Build history of the part. All positions in model axes, mm. Face numbers are marked on the shaded views. A direction names the side the tool comes from. Give positions to 0.01 mm unless a question says otherwise; leave off trailing zeros. Order: outer loops, then holes, each group sorted by start corner. A loop starts at its lowest first (then second) coordinate and runs counter-clockwise, first axis right, second up. Notation, with made-up numbers: (81, 23) - (97, 23) arc R33 ccw to (97, 56) - close; hole circle Ø8 at (33, 7). An arc over 180 degrees is marked (long way). Use a Markdown table: item, result. Add a question column.
(1) Flat gauge pins, fed straight in: pin 1 (6 mm diameter, centred on x = -6.5, z = 0, fed in from +Y); pin 2 (0.6 mm diameter, centred on x = 17.5, y = 2.5, fed in from +Z); pin 3 (1.2 mm diameter, centred on x = -20.75, z = -7.75, fed in from -Y); pin 4 (1.6 mm diameter, centred on x = 20.5, y = 4.5, fed in from -Z). Where does each tip first touch, or does it go through?
(2) Slice it at A-A (z = 7.75). Write the cut outline in (x, y).
(3) Wall check: line 1 (Z direction, x = 20.75, y = 1.25); line 2 (X direction, y = 0.35, z = 7.75); line 3 (Y direction, x = -18.5, z = 3.5). Give the ranges that are in metal, low to high.
(4) Slice it at B-B (x = -20.75). Write the cut outline in (y, z), then the cut area to 3 significant figures.
(5) Slice it at D-D (z = 1.5). Write the cut outline in (x, y), then the cut area to 3 significant figures.
(6) Which spindle directions (+Z, -Z, +X, -X, +Y, -Y) get a long thin tool onto all of the face, cutting with end or side? Do the marked faces 1 and 2. Say none if no direction does.
(7) Slice it at C-C (x = 16). Write the cut outline in (y, z), then the cut area to 3 significant figures.
from build123d import *

# Parameters (mm, degrees)
SCHIZZO1_W                   = 44
SCHIZZO1_H                   = 18
ESTRUSIONE_ESTRUSIONE1_DEPTH = 1.5
SCHIZZO2_R                   = 0.75
TAGLIO_ESTRUSIONE1_DEPTH     = 1.5
SCHIZZO4_W                   = 10
SCHIZZO4_H                   = 7
ESTRUSIONE_ESTRUSIONE2_DEPTH = 2
SCHIZZO5_W                   = 10
SCHIZZO5_H                   = 8
ESTRUSIONE_ESTRUSIONE3_DEPTH = 2


with BuildPart() as part:
    # Schizzo1 → Estrusione-Estrusione1 (new body)
    with BuildSketch(Plane(origin=(0, 0, 0), x_dir=(1, 0, 0), z_dir=(0, 1, 0))):
        Rectangle(SCHIZZO1_W, SCHIZZO1_H)
    extrude(amount=ESTRUSIONE_ESTRUSIONE1_DEPTH)

    # Schizzo2 → Taglio-Estrusione1 (cut)
    with BuildSketch(Plane(origin=(0, 1.5, 0), x_dir=(1, 0, 0), z_dir=(0, 1, 0))):
        with Locations((-20.75, 7.75)):
            Circle(SCHIZZO2_R)
        with Locations((20.75, 7.75)):
            Circle(SCHIZZO2_R)
        with Locations((20.75, -7.75)):
            Circle(SCHIZZO2_R)
        with Locations((-20.75, -7.75)):
            Circle(SCHIZZO2_R)
    extrude(amount=-TAGLIO_ESTRUSIONE1_DEPTH, mode=Mode.SUBTRACT)

    # Schizzo4 → Estrusione-Estrusione2 (add)
    with BuildSketch(Plane(origin=(0, 1.5, 0), x_dir=(1, 0, 0), z_dir=(0, 1, 0))):
        with Locations((19, 0)):
            Rectangle(SCHIZZO4_W, SCHIZZO4_H)
    extrude(amount=ESTRUSIONE_ESTRUSIONE2_DEPTH)

    # Schizzo5 → Estrusione-Estrusione3 (add)
    with BuildSketch(Plane(origin=(0, 3.5, 0), x_dir=(1, 0, 0), z_dir=(0, 1, 0))):
        with Locations((19, 0)):
            Rectangle(SCHIZZO5_W, SCHIZZO5_H)
    extrude(amount=ESTRUSIONE_ESTRUSIONE3_DEPTH)


solid = part.part
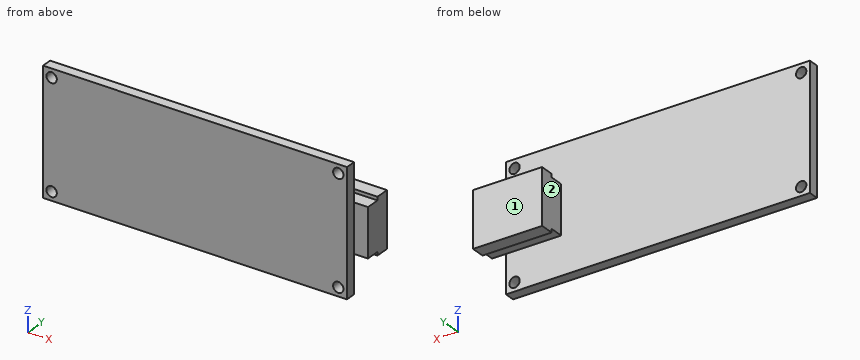
Solution:
| question | item | result |
|---|---|---|
| 1 | pin 1 | y = 1.5 |
| 1 | pin 2 | z = 3.5 |
| 1 | pin 3 | through |
| 1 | pin 4 | z = -4 |
| 2 | outline | (-22, 0) - (-21.5, 0) - (-21.5, 1.5) - (-22, 1.5) - close; (-20, 0) - (20, 0) - (20, 1.5) - (-20, 1.5) - close; (21.5, 0) - (22, 0) - (22, 1.5) - (21.5, 1.5) - close |
| 3 | line 1 | -9 to -8.5, -7 to 7, 8.5 to 9 |
| 3 | line 2 | -22 to -21.5, -20 to 20, 21.5 to 22 |
| 3 | line 3 | 0 to 1.5 |
| 4 | outline | (0, -9) - (1.5, -9) - (1.5, -8.5) - (0, -8.5) - close; (0, -7) - (1.5, -7) - (1.5, 7) - (0, 7) - close; (0, 8.5) - (1.5, 8.5) - (1.5, 9) - (0, 9) - close |
| 4 | area | 22.5 mm2 |
| 5 | outline | (-22, 0) - (22, 0) - (22, 1.5) - (24, 1.5) - (24, 5.5) - (14, 5.5) - (14, 1.5) - (-22, 1.5) - close |
| 5 | area | 106 mm2 |
| 6 | face 1 | +Z, -Z, +X, -X, +Y |
| 6 | face 2 | +Z, -Z, -X, +Y |
| 7 | outline | (0, -9) - (1.5, -9) - (1.5, -3.5) - (3.5, -3.5) - (3.5, -4) - (5.5, -4) - (5.5, 4) - (3.5, 4) - (3.5, 3.5) - (1.5, 3.5) - (1.5, 9) - (0, 9) - close |
| 7 | area | 57.0 mm2 |
